Geometry check sheet. Reference: drawing and pictorial views, mm from the part's lowest x, y, z. A direction names the side the tool comes from. Coordinates: 2 decimals unless noted, no trailing zeros. Loops run counter-clockwise (first coordinate to the right, second up) from the corner with the lowest first, then second, coordinate; pieces in that order, holes last. Notation, with made-up numbers: (29.25, -16) - (52.25, -16) arc R18 ccw to (52.25, 12) - close; hole circle Ø5 at (22, 80). An arc over 180 degrees is marked (long way). Use a Markdown table: item, result. Add a question column.
1) Sectioned sample at A-A, the plane y = 175. Enter the section's corners in (x, z).
2) Sectioned sample at D-D, the plane x = 13.5. Enter the section's corners in (y, z), then the cut area to 3 significant figures.
3) Sectioned sample at C-C, the plane z = 6.25. Enter the section's corners in (x, y), then the cut area to 3 significant figures.
4) Go/stop test with flat-tipped pins: P1, Ø11, axis at y = 173.5, z = 8, coming from the +X side; P2, Ø8, axis at x = 84.5, y = 150, coming from the +Z side; P3, Ø11, axis at y = 235, z = 9, coming from the +X side; P4, Ø5, axis at y = 174, z = 9, coming from the -X side. Record where each tip stops, or that it passes through.
5) Sectioned sample at B-B, the plane x = 50. Enter the section's corners in (y, z), then the cut area to 3 significant figures.
6) Thickness scan on line 1 (Y direction, x = 50, z = 11.75); line 2 (Y direction, x = 16.5, z = 19); line 3 (Y direction, x = 145.5, z = 15). Record the ranges inside material, lowest first.
7) Tool access check on the marked faces 1 and 2. Record the directions out of +Z, -Z, +X, -X, +Y, -Y that give a thin tool (end or side, any length) a straight path to the whole face; none if there is none.
8) Draft check along X on the marked faces 3, 4 and 5. Enter one of: pulls with the +X half, pulls with the -X half, needs draft (parallel to the pull), parting line crosses it, or undercut.
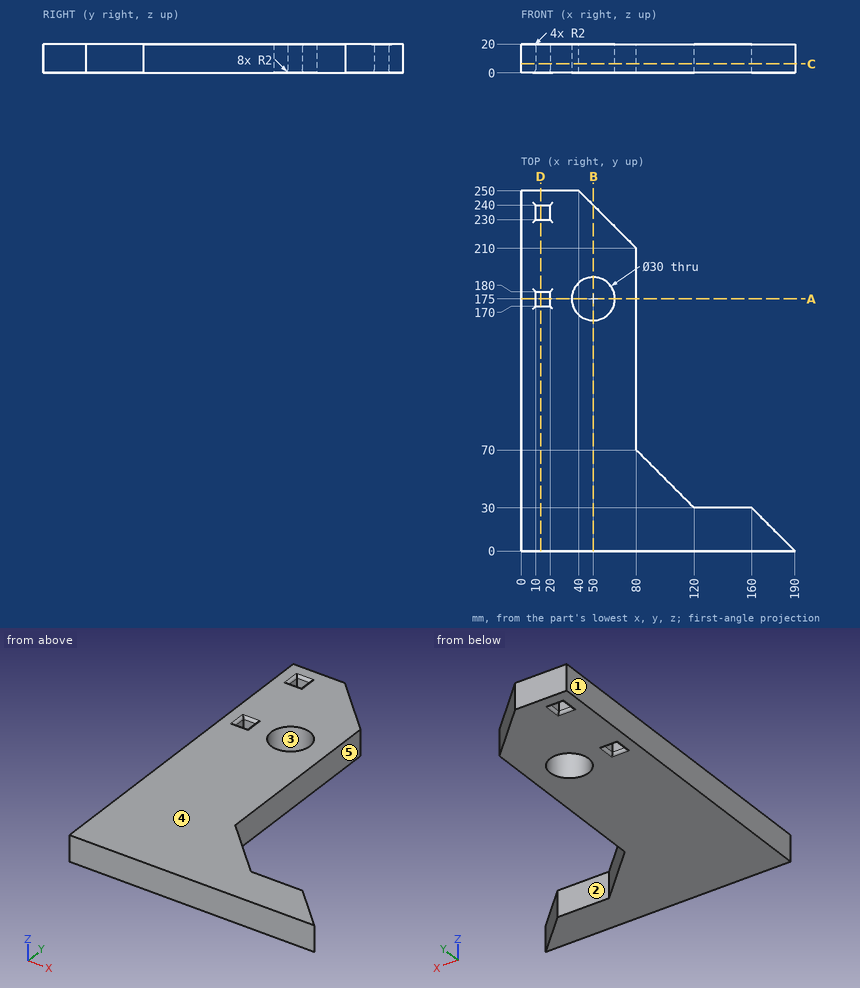
Solved:
| question | item | result |
|---|---|---|
| 1 | outline | (0, 0) - (8, 0) arc R2 ccw to (10, 2) - (10, 18) arc R2 ccw to (8, 20) - (0, 20) - close; (20, 2) arc R2 ccw to (22, 0) - (35, 0) - (35, 20) - (22, 20) arc R2 ccw to (20, 18) - close; (65, 0) - (80, 0) - (80, 20) - (65, 20) - close |
| 2 | outline | (0, 0) - (168, 0) arc R2 ccw to (170, 2) - (170, 18) arc R2 ccw to (168, 20) - (0, 20) - close; (180, 2) arc R2 ccw to (182, 0) - (228, 0) arc R2 ccw to (230, 2) - (230, 18) arc R2 ccw to (228, 20) - (182, 20) arc R2 ccw to (180, 18) - close; (240, 2) arc R2 ccw to (242, 0) - (250, 0) - (250, 20) - (242, 20) arc R2 ccw to (240, 18) - close |
| 2 | area | 4,590 mm2 |
| 3 | outline | (0, 0) - (190, 0) - (160, 30) - (120, 30) - (80, 70) - (80, 210) - (40, 250) - (0, 250) - close; hole (10, 170) - (20, 170) - (20, 180) - (10, 180) - close; hole (10, 230) - (20, 230) - (20, 240) - (10, 240) - close; hole circle Ø30 at (50, 175) |
| 3 | area | 21,900 mm2 |
| 4 | P1 | stops at x = 80 |
| 4 | P2 | passes through |
| 4 | P3 | stops at x = 60.5 |
| 4 | P4 | stops at x = 0 |
| 5 | outline | (0, 0) - (160, 0) - (160, 20) - (0, 20) - close; (190, 0) - (240, 0) - (240, 20) - (190, 20) - close |
| 5 | area | 4,200 mm2 |
| 6 | line 1 | y = 0 to 160, 190 to 240 |
| 6 | line 2 | y = 0 to 169.73, 180.27 to 229.73, 240.27 to 250 |
| 6 | line 3 | y = 0 to 30 |
| 7 | face 1 | +Z, -Z, -X, +Y, -Y |
| 7 | face 2 | +Z, -Z, +X, +Y |
| 8 | face 3 | undercut |
| 8 | face 4 | needs draft |
| 8 | face 5 | pulls with the +X half |
